Part model, mm, in its own coordinate system. Round coordinates to 2 decimals unless told otherwise and drop trailing zeros. Write each loop counter-clockwise with the first axis right and the second up, starting at its lowest first coordinate (ties: lowest second). Pieces come first, ordered by that corner, then holes. Notation, with made-up numbers: M 52,-4 L 110,-4 A27 cw 110,14 Z; hole C 17.5,54.5 d2. An arc over 180 degrees is marked long. Use one line per item in the form item = value. Start each with the question number.
Item 1: Cut at C-C, the plane z = 0. Give the cut face in (x, y).
Item 2: Cut at A-A, the plane x = -80.5. Give the cut face in (y, z).
Item 3: Cut at B-B, the plane y = 0.9. Give the cut face in (x, z).
Item 4: Probe L1, parallel to X at y = 2.35, z = 2.5; L2, parallel to X at y = 1.2, z = -3.25; L3, parallel to Z at x = 96, y = 2.5. List the from-to ranges inside material, lowest first.
Item 5: Cut at D-D, the plane x = 99. Give the cut face in (y, z), then the cut area to 3 significant figures.
Item 6: Flat gauge pins, fed straight in: pin 1 Ø4 at (x, z) = (80.5, 0) entering from -Y; pin 2 Ø11 at (x, z) = (-99, 0) entering from -Y. Where does each tip first touch, or does it go through?
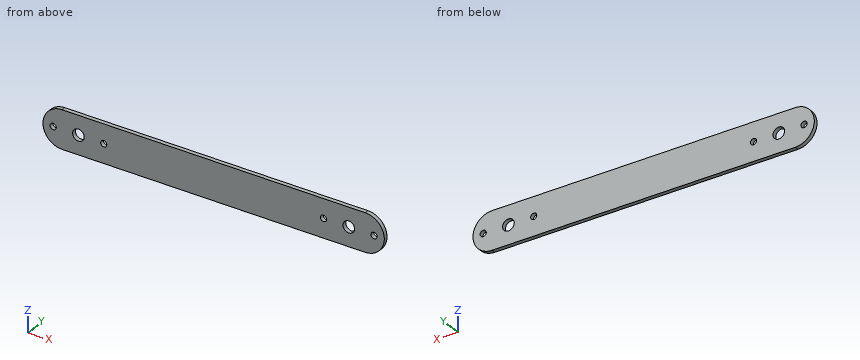
from build123d import *

# Parameters (mm, degrees)
SKETCH_1_W          = 250
SKETCH_1_H          = 28
EXTRUDE_1_DEPTH     = 3
CUT_EXTRUDE_1_REACH = 127.817
SKETCH_2_R          = 4.25
CUT_EXTRUDE_2_REACH = 127.817
SKETCH_3_R          = 2.25
FILLET_1_RADIUS     = 14
FILLET_1_LENGTH     = 3
FILLET_2_RADIUS     = 14
FILLET_2_LENGTH     = 3


with BuildPart() as part:
    # 草图1 → 凸台-拉伸1 (new body)
    with BuildSketch(Plane(origin=(0, 0, 0), x_dir=(1, 0, 0), z_dir=(0, 1, 0))):
        Rectangle(SKETCH_1_W, SKETCH_1_H)
    extrude(amount=EXTRUDE_1_DEPTH)

    # 草图2 → 切除-拉伸1 (cut, up to next)
    with BuildSketch(Plane(origin=(0, 3, 0), x_dir=(1, 0, 0), z_dir=(0, 1, 0)), mode=Mode.PRIVATE) as cut_extrude_1_sk1:
        with Locations(Location((-99, 0, 0), (0, 0, 270))):
            Circle(SKETCH_2_R)
    cut_extrude_1_tool1 = extrude(cut_extrude_1_sk1.sketch, amount=-CUT_EXTRUDE_1_REACH, mode=Mode.PRIVATE) & part.part
    # 草图2 → 切除-拉伸1 (cut, up to next)
    with BuildSketch(Plane(origin=(0, 3, 0), x_dir=(1, 0, 0), z_dir=(0, 1, 0)), mode=Mode.PRIVATE) as cut_extrude_1_sk2:
        with Locations(Location((99, 0, 0), (0, 0, 270))):
            Circle(SKETCH_2_R)
    cut_extrude_1_tool2 = extrude(cut_extrude_1_sk2.sketch, amount=-CUT_EXTRUDE_1_REACH, mode=Mode.PRIVATE) & part.part
    add(cut_extrude_1_tool1.solids().sort_by_distance((-99, 3, 0))[0], mode=Mode.SUBTRACT)
    add(cut_extrude_1_tool2.solids().sort_by_distance((99, 3, 0))[0], mode=Mode.SUBTRACT)

    # 草图3 → 切除-拉伸2 (cut, up to next)
    with BuildSketch(Plane(origin=(0, 3, 0), x_dir=(1, 0, 0), z_dir=(0, 1, 0)), mode=Mode.PRIVATE) as cut_extrude_2_sk1:
        with Locations(Location((-117.5, 0, 0), (0, 0, 270))):
            Circle(SKETCH_3_R)
    cut_extrude_2_tool1 = extrude(cut_extrude_2_sk1.sketch, amount=-CUT_EXTRUDE_2_REACH, mode=Mode.PRIVATE) & part.part
    # 草图3 → 切除-拉伸2 (cut, up to next)
    with BuildSketch(Plane(origin=(0, 3, 0), x_dir=(1, 0, 0), z_dir=(0, 1, 0)), mode=Mode.PRIVATE) as cut_extrude_2_sk2:
        with Locations(Location((-80.5, 0, 0), (0, 0, 270))):
            Circle(SKETCH_3_R)
    cut_extrude_2_tool2 = extrude(cut_extrude_2_sk2.sketch, amount=-CUT_EXTRUDE_2_REACH, mode=Mode.PRIVATE) & part.part
    # 草图3 → 切除-拉伸2 (cut, up to next)
    with BuildSketch(Plane(origin=(0, 3, 0), x_dir=(1, 0, 0), z_dir=(0, 1, 0)), mode=Mode.PRIVATE) as cut_extrude_2_sk3:
        with Locations(Location((80.5, 0, 0), (0, 0, 270))):
            Circle(SKETCH_3_R)
    cut_extrude_2_tool3 = extrude(cut_extrude_2_sk3.sketch, amount=-CUT_EXTRUDE_2_REACH, mode=Mode.PRIVATE) & part.part
    # 草图3 → 切除-拉伸2 (cut, up to next)
    with BuildSketch(Plane(origin=(0, 3, 0), x_dir=(1, 0, 0), z_dir=(0, 1, 0)), mode=Mode.PRIVATE) as cut_extrude_2_sk4:
        with Locations(Location((117.5, 0, 0), (0, 0, 270))):
            Circle(SKETCH_3_R)
    cut_extrude_2_tool4 = extrude(cut_extrude_2_sk4.sketch, amount=-CUT_EXTRUDE_2_REACH, mode=Mode.PRIVATE) & part.part
    add(cut_extrude_2_tool1.solids().sort_by_distance((-117.5, 3, 0))[0], mode=Mode.SUBTRACT)
    add(cut_extrude_2_tool2.solids().sort_by_distance((-80.5, 3, 0))[0], mode=Mode.SUBTRACT)
    add(cut_extrude_2_tool3.solids().sort_by_distance((80.5, 3, 0))[0], mode=Mode.SUBTRACT)
    add(cut_extrude_2_tool4.solids().sort_by_distance((117.5, 3, 0))[0], mode=Mode.SUBTRACT)

    # 圆角1: full round fillet: the end face becomes a half cylinder, R = half its width
    fillet_1_face = Plane((-125, 1.5, 0), x_dir=(0, 1, 0), z_dir=(-1, 0, 0))  # on the end face: x along it, z out of the body
    fillet_1_slab = fillet_1_face.offset(-FILLET_1_RADIUS / 2) * Box(FILLET_1_LENGTH, 2 * FILLET_1_RADIUS, FILLET_1_RADIUS, mode=Mode.PRIVATE)  # the body's end, R deep
    fillet_1_round = Plane((-111, 1.5, 0), x_dir=(-1, 0, 0), z_dir=(0, 1, 0)) * Cylinder(FILLET_1_RADIUS, FILLET_1_LENGTH, mode=Mode.PRIVATE)  # its axis R under the face
    add(fillet_1_slab - fillet_1_round, mode=Mode.SUBTRACT)

    # 圆角2: full round fillet: the end face becomes a half cylinder, R = half its width
    fillet_2_face = Plane((125, 1.5, 0), x_dir=(0, -1, 0), z_dir=(1, 0, 0))  # on the end face: x along it, z out of the body
    fillet_2_slab = fillet_2_face.offset(-FILLET_2_RADIUS / 2) * Box(FILLET_2_LENGTH, 2 * FILLET_2_RADIUS, FILLET_2_RADIUS, mode=Mode.PRIVATE)  # the body's end, R deep
    fillet_2_round = Plane((111, 1.5, 0), x_dir=(1, 0, 0), z_dir=(0, -1, 0)) * Cylinder(FILLET_2_RADIUS, FILLET_2_LENGTH, mode=Mode.PRIVATE)  # its axis R under the face
    add(fillet_2_slab - fillet_2_round, mode=Mode.SUBTRACT)


solid = part.part
Model answer:
q1.outline = M -125,0 L -119.75,0 L -119.75,3 L -125,3 Z; M -115.25,0 L -103.25,0 L -103.25,3 L -115.25,3 Z; M -94.75,0 L -82.75,0 L -82.75,3 L -94.75,3 Z; M -78.25,0 L 78.25,0 L 78.25,3 L -78.25,3 Z; M 82.75,0 L 94.75,0 L 94.75,3 L 82.75,3 Z; M 103.25,0 L 115.25,0 L 115.25,3 L 103.25,3 Z; M 119.75,0 L 125,0 L 125,3 L 119.75,3 Z
q2.outline = M 0,-14 L 3,-14 L 3,-2.25 L 0,-2.25 Z; M 0,2.25 L 3,2.25 L 3,14 L 0,14 Z
q3.outline = M -111,-14 L 111,-14 A14 ccw 111,14 L -111,14 A14 ccw Z; hole C -117.5,0 d4.5; hole C -99,0 d8.5; hole C -80.5,0 d4.5; hole C 80.5,0 d4.5; hole C 99,0 d8.5; hole C 117.5,0 d4.5
q4.L1 = -124.77 to -102.44, -95.56 to 95.56, 102.44 to 124.77
q4.L2 = -124.62 to -101.74, -96.26 to 96.26, 101.74 to 124.62
q4.L3 = -14 to -3.01, 3.01 to 14
q5.outline = M 0,-14 L 3,-14 L 3,-4.25 L 0,-4.25 Z; M 0,4.25 L 3,4.25 L 3,14 L 0,14 Z
q5.area = 58.5 mm²
q6.pin_1 = through
q6.pin_2 = 0
